Design review of the part built by this model. Coordinates are the model's own, in mm. Round coordinates to 2 decimals unless told otherwise and drop trailing zeros. Order: outer loops, then holes, each group sorted by start corner. A loop starts at its lowest first (then second) coordinate and runs counter-clockwise, first axis right, second up. Notation, with made-up numbers: (82.5, 3) - (96.5, 3) arc R29 ccw to (96.5, 24) - close; hole circle Ø6 at (2.25, -3.75). An arc over 180 degrees is marked (long way). Answer as a JSON object with one key per item and string values. Group by question number.
Autodesk Inventor part; units mm, degrees
ref_plane "YZ Plane" through (0, 0, 0) normal (1, 0, 0) x (0, 1, 0)
ref_plane "XZ Plane" through (0, 0, 0) normal (0, 1, 0) x (-1, 0, 0)
ref_plane "XY Plane" through (0, 0, 0) normal (0, 0, 1) x (1, 0, 0)
sketch "Эскиз1" plane through (0, 0, 0) normal (0, 1, 0) x (-1, 0, 0)
  circle A0 centre (0, 0) radius 85
  circle A1 centre (0, 0) radius 4
  dimension "d0" = 170
  dimension "d15" = 8
extrude "Выдавливание1" add sketch "Эскиз1" along normal blind 6
sketch "Эскиз2" plane through (0, 0, 0) normal (0, -1, 0) x (1, 0, 0)
  circle A0 centre (0, 0) radius 4
  circle A1 centre (0, 0) radius 117.5181 construction
  line L0 (101.7737, 58.7591) -> (0, -117.5181) construction
  line L1 (0, -117.5181) -> (-101.7737, 58.7591) construction
  line L2 (-101.7737, 58.7591) -> (101.7737, 58.7591) construction
  line L3 (16.15, 64.9091) -> (-16.15, 64.9091)
  line L4 (-16.15, 64.9091) -> (-16.15, 52.6091)
  line L5 (-16.15, 52.6091) -> (16.15, 52.6091)
  line L6 (16.15, 52.6091) -> (16.15, 64.9091)
  line L7 (16.15, 64.9091) -> (-16.15, 52.6091) construction
  line L8 (-16.15, 64.9091) -> (16.15, 52.6091) construction
  line L9 (-16.15, 58.7591) -> (16.15, 58.7591) construction
  line L10 (-64.2879, -18.4682) -> (-48.1379, -46.4408)
  line L11 (-37.4858, -40.2908) -> (-53.6358, -12.3182)
  line L12 (-53.6358, -12.3182) -> (-64.2879, -18.4682)
  line L13 (-48.1379, -46.4408) -> (-37.4858, -40.2908)
  line L14 (-64.2879, -18.4682) -> (-37.4858, -40.2908) construction
  line L15 (-48.1379, -46.4408) -> (-53.6358, -12.3182) construction
  line L16 (48.1379, -46.4408) -> (64.2879, -18.4682)
  line L17 (53.6358, -12.3182) -> (37.4858, -40.2908)
  line L18 (37.4858, -40.2908) -> (48.1379, -46.4408)
  line L19 (64.2879, -18.4682) -> (53.6358, -12.3182)
  line L20 (48.1379, -46.4408) -> (53.6358, -12.3182) construction
  line L21 (64.2879, -18.4682) -> (37.4858, -40.2908) construction
  circle A2 centre (58.0718, 25.9871) radius 6
  circle A3 centre (18.6407, 0) radius 2.5
  circle A4 centre (-18.3593, 0) radius 2.5
  point P0 (0, 58.7591)
  point P1 (-58.9618, -15.3932)
  point P2 (-42.8118, -43.3658)
  point P3 (-50.8868, -29.3795)
  point P4 (42.8118, -43.3658)
  point P5 (58.9618, -15.3932)
  point P6 (50.8868, -29.3795)
  dimension "d16" = 32.3
  dimension "d17" = 12.3
  dimension "d20" = 360
  dimension "d25" = 12
  dimension "d26" = 5
  dimension "d27" = 5
  dimension "d28" = 37
extrude "Выдавливание3" cut sketch "Эскиз2" against normal blind 6 contours L6 L5 L4 L3 | L12 L11 L13 L10 | L18 L17 L19 L16 | A2 | A3 | A4
sketch "Эскиз3" plane through (0, 0, 0) normal (0, -1, 0) x (1, 0, 0)
  point P0 (0, 0)
sketch "Эскиз4" plane through (0, 0, 0) normal (0, -1, 0) x (1, 0, 0)
  point P0 (0, 0)
sketch "Эскиз5" plane through (0, 0, 0) normal (0, -1, 0) x (1, 0, 0)
  circle A0 centre (65.8248, 32.4068) radius 1.25 construction
  circle A1 centre (73.5684, 18.9798) radius 1.25 construction
  circle A2 centre (50.3248, 32.4142) radius 1.25 construction
  circle A3 centre (65.8121, 5.5601) radius 1.25 construction
  circle A4 centre (61.3843, 6.6933) radius 1.19 construction
  circle A5 centre (65.8121, 5.5601) radius 1.25 construction
  circle A6 centre (50.3121, 5.5674) radius 1.25 construction
  circle A7 centre (42.5684, 18.9944) radius 1.25 construction
  circle A8 centre (50.3248, 32.4142) radius 1.25 construction
  circle A9 centre (73.5684, 18.9798) radius 1.5
  circle A10 centre (65.8121, 5.5601) radius 1.5
  circle A11 centre (50.3121, 5.5674) radius 1.5
  circle A12 centre (42.5684, 18.9944) radius 1.5
  circle A13 centre (50.3248, 32.4142) radius 1.5
  circle A14 centre (65.8248, 32.4068) radius 1.5
  point P0 (0, 0)
  dimension "d29" = 3
  dimension "d30" = 3
  dimension "d31" = 3
  dimension "d32" = 3
  dimension "d33" = 3
  dimension "d34" = 3
extrude "Выдавливание4" cut sketch "Эскиз5" against normal blind 10
sketch "Эскиз6" plane through (0, 0, 0) normal (0, -1, 0) x (1, 0, 0)
  circle A0 centre (-59.3361, -10.0795) radius 1.65
  circle A1 centre (-38.3361, -46.4526) radius 1.65
  circle A2 centre (38.6083, -46.4687) radius 1.65
  circle A3 centre (59.6083, -10.0956) radius 1.65
  circle A4 centre (21.15, 56.5482) radius 1.65
  circle A5 centre (-20.85, 56.5482) radius 1.65
  point P0 (0, 0)
extrude "Выдавливание5" cut sketch "Эскиз6" against normal blind 10
sketch "Эскиз10" plane through (0, 0, 0) normal (0, -1, 0) x (1, 0, 0)
  line L0 (29.5, 68.4725) -> (32.5, 68.4725)
  line L1 (29.5, 58.4725) -> (29.5, 68.4725)
  line L2 (32.5, 58.4725) -> (29.5, 58.4725)
  line L3 (32.5, 68.4725) -> (32.5, 58.4725)
  line L4 (29.5, 48.4725) -> (32.5, 48.4725)
  line L5 (29.5, 38.4725) -> (29.5, 48.4725)
  line L6 (32.5, 38.4725) -> (29.5, 38.4725)
  line L7 (32.5, 48.4725) -> (32.5, 38.4725)
  line L8 (29.5, 18.4725) -> (32.5, 18.4725)
  line L9 (29.5, 8.4725) -> (29.5, 18.4725)
  line L10 (32.5, 8.4725) -> (29.5, 8.4725)
  line L11 (32.5, 18.4725) -> (32.5, 8.4725)
  line L12 (29.5, -1.5275) -> (32.5, -1.5275)
  line L13 (29.5, -11.5275) -> (29.5, -1.5275)
  line L14 (32.5, -11.5275) -> (29.5, -11.5275)
  line L15 (32.5, -1.5275) -> (32.5, -11.5275)
  line L16 (-29.5, -1.5275) -> (-32.5, -1.5275)
  line L17 (-32.5, -1.5275) -> (-32.5, -11.5275)
  line L18 (-32.5, -11.5275) -> (-29.5, -11.5275)
  line L19 (-29.5, -11.5275) -> (-29.5, -1.5275)
  line L20 (-29.5, 18.4725) -> (-32.5, 18.4725)
  line L21 (-32.5, 18.4725) -> (-32.5, 8.4725)
  line L22 (-32.5, 8.4725) -> (-29.5, 8.4725)
  line L23 (-29.5, 8.4725) -> (-29.5, 18.4725)
  line L24 (-29.5, 48.4725) -> (-32.5, 48.4725)
  line L25 (-32.5, 48.4725) -> (-32.5, 38.4725)
  line L26 (-32.5, 38.4725) -> (-29.5, 38.4725)
  line L27 (-29.5, 38.4725) -> (-29.5, 48.4725)
  line L28 (-29.5, 68.4725) -> (-32.5, 68.4725)
  line L29 (-32.5, 68.4725) -> (-32.5, 58.4725)
  line L30 (-32.5, 58.4725) -> (-29.5, 58.4725)
  line L31 (-29.5, 58.4725) -> (-29.5, 68.4725)
  circle A0 centre (-31, 53.4725) radius 1.5
  circle A1 centre (-31, 3.4725) radius 1.5
  circle A2 centre (31, 53.4725) radius 1.5
  circle A3 centre (31, 3.4725) radius 1.5
  line L32 (-31, 58.4725) -> (-31, 48.4725) construction
  line L33 (-31, 8.4725) -> (-31, -1.5275) construction
  line L34 (31, -1.5275) -> (31, 8.4725) construction
  line L35 (31, 48.4725) -> (31, 58.4725) construction
  point P0 (0, 0)
  point P1 (-31, 53.4725)
  point P2 (-31, 3.4725)
  point P3 (31, 3.4725)
  dimension "d57" = 3
extrude "Выдавливание9" cut sketch "Эскиз10" against normal up to surface (6 mm away)
properties part number "Fanerka"
1. Clearance check with flat-ended pins moving along their axes: P1, Ø3, axis at y = 4.5, z = 49, coming from the +X side; P2, Ø1.5, axis at x = -7.5, y = 5, coming from the +Z side; P3, Ø1.5, axis at x = -30.5, y = 3, coming from the +Z side; P4, Ø1.8, axis at x = 73.57, z = 18.98, coming from the -Y side. State where each tip first meets the part, or that it passes through.
2. To check wall thickness, follow line 1 (Z direction, x = 60, y = 0.75); line 2 (X direction, y = 3.65, z = -34.5); line 3 (X direction, y = 4.2, z = -12.5). State the ranges of each line that lie inside material, in increasing order. Write a range as from..to.
3. Take a section at D-D, the plane x = -26. Give the boundary of the cut face in (y, z), then the cut area to 3 significant figures.
4. Take a section at A-A, the plane x = 0. Give the boundary of the cut face in (y, z).
5. Take a section at C-C, the plane y = 2.35. Count the separate pieces of the cut face and the enclosed holes in it, then the cut area to 3 significant figures.
6. Take a section at B-B, the plane z = -30.5. Give the boundary of the cut face in (x, y), then the cut area to 3 significant figures.
7. Mouldability with a two-part tool opening along X and no side actions: class faces 1 (the cylindrical face through (67.453, 2.958, 51.721)), 2 (the flat face through (42.7, 3, -43.3)), 3 (the flat face through (1, 6, -18)) as pulls with the +X half, pulls with the -X half, needs draft (parallel to the pull), parting line crosses it, or undercut.
Response values:
{
 "1": {"P1": "x = 70.49", "P2": "z = 84.73", "P3": "z = 79.62", "P4": "through"},
 "2": {"line 1": "-60.21..-25.9, -15.99..-11.7, -8.49..20.31, 31.67..60.21", "line 2": "-77.68..-55.03, -40.83..40.83, 55.03..77.68", "line 3": "-84.08..-53.95, -53.53..53.53, 53.95..84.08"},
 "3": {"outline": "(0, -80.93) - (6, -80.93) - (6, 80.93) - (0, 80.93) - close", "area": "971 mm2"},
 "4": {"outline": "(0, -85) - (6, -85) - (6, -4) - (0, -4) - close; (0, 4) - (6, 4) - (6, 52.61) - (0, 52.61) - close; (0, 64.91) - (6, 64.91) - (6, 85) - (0, 85) - close"},
 "5": {"separate pieces": "1", "enclosed holes": "31", "area": "20,900 mm2"},
 "6": {"outline": "(-79.34, 0) - (-57.34, 0) - (-57.34, 6) - (-79.34, 6) - close; (-43.14, 0) - (43.14, 0) - (43.14, 6) - (-43.14, 6) - close; (57.34, 0) - (79.34, 0) - (79.34, 6) - (57.34, 6) - close", "area": "782 mm2"},
 "7": {"face 1": "parting line crosses it", "face 2": "undercut", "face 3": "needs draft"}
}
